Geometry: see drawing. Coordinates: mm, zero at the bounding-box minimum. Coordinates: 2 decimals unless noted, no trailing zeros. Order: outer loops, then holes, each group sorted by start corner. A loop starts at its lowest first (then second) coordinate and runs counter-clockwise, first axis right, second up.
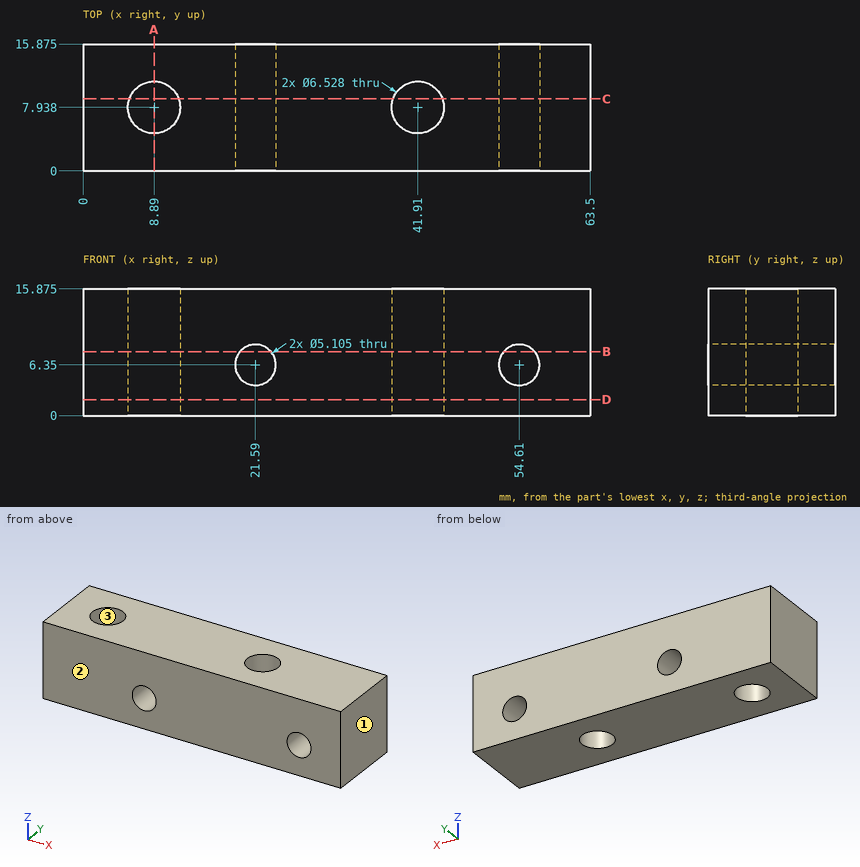
Q1. Section query C-C on y = 9. Give the number of separate pieces and of enclosed holes in the cut face, plus the area to 3 significant figures.
Solutions:
separate pieces: 3
enclosed holes: 2
area: 771 mm2
Q2. Material intervals for line 1 along Z through (x, y) = (21.59, 7.25) (1 decimal); line 2 along X through (y, z) = (8.5, 13) (1 decimal); line 3 along X through (y, z) = (1.25, 8), sorted ascending.
Solutions:
line 1: z = 0 to 3.8, 8.9 to 15.9
line 2: x = 0 to 5.7, 12.1 to 38.7, 45.1 to 63.5
line 3: x = 0 to 19.64, 23.54 to 52.66, 56.56 to 63.5
Q3. Section query D-D on z = 2. Output: boundary loops of the cut face in (x, y) (1 decimal), plus the area to 3 significant figures.
Solutions:
outline: (0, 0) - (63.5, 0) - (63.5, 15.9) - (0, 15.9) - close; hole circle Ø6.5 at (8.9, 7.9); hole circle Ø6.5 at (41.9, 7.9)
area: 941 mm2
Q4. Pull-direction query (Y, two-part tool) for the marked faces 1, 2 and 3; classes: pulls with the +Y half, pulls with the -Y half, needs draft (parallel to the pull), parting line crosses it, or undercut.
Solutions:
face 1: needs draft
face 2: pulls with the -Y half
face 3: undercut
Q5. Section query A-A on x = 8.89. Output: boundary loops of the cut face in (y, z) (1 decimal), plus the area to 3 significant figures.
Solutions:
outline: (0, 0) - (4.7, 0) - (4.7, 15.9) - (0, 15.9) - close; (11.2, 0) - (15.9, 0) - (15.9, 15.9) - (11.2, 15.9) - close
area: 148 mm2
Q6. Section query B-B on z = 8. Output: boundary loops of the cut face in (x, y) (1 decimal).
Solutions:
outline: (0, 0) - (19.6, 0) - (19.6, 15.9) - (0, 15.9) - close; (23.5, 0) - (52.7, 0) - (52.7, 15.9) - (23.5, 15.9) - close; (56.6, 0) - (63.5, 0) - (63.5, 15.9) - (56.6, 15.9) - close; hole circle Ø6.5 at (8.9, 7.9); hole circle Ø6.5 at (41.9, 7.9)
